from build123d import *
from build123d.topology import SkipClean

# Parameters (mm, degrees)
SKETCH1_R                 = 1.5
BOSS_EXTRUDE1_DEPTH       = 5
BOSS_EXTRUDE3_DEPTH       = 5
SKETCH4_R                 = 2.5
CUT_EXTRUDE2_DEPTH        = 5
BOSS_EXTRUDE4_DEPTH       = 5
BOSS_EXTRUDE4_2_DEPTH     = 5
BOSS_EXTRUDE5_OUTLINE_R   = 2.5
BOSS_EXTRUDE5_OUTLINE_R_2 = 1.5
BOSS_EXTRUDE5_DEPTH       = 0.01
CUT_EXTRUDE3_DEPTH        = 10
SKETCH10_R                = 1.5
CUT_EXTRUDE4_DEPTH        = 10


# Read off the part's stored shape, not the designer's step: Boss-Extrude5
with BuildPart() as part:
    # Sketch1 → Boss-Extrude1 (new body)
    with BuildSketch(Plane.XY):
        with BuildLine():
            Line((0, -4), (-70.14, -4))
            ThreePointArc((-70.14, -4), (-74.14, 0), (-70.14, 4))
            Line((-70.14, 4), (0, 4))
            ThreePointArc((0, 4), (4, 0), (0, -4))
        make_face()
        with Locations((-70.14, 0)):
            Circle(SKETCH1_R, mode=Mode.SUBTRACT)
        Circle(SKETCH1_R, mode=Mode.SUBTRACT)
    extrude(amount=BOSS_EXTRUDE1_DEPTH)

    # Sketch3 → Boss-Extrude3 (add)
    with BuildSketch(Plane.XY):
        with BuildLine():
            Line((-70.14, -4), (-77.64, -4))
            ThreePointArc((-77.64, -4), (-81.64, 0), (-77.64, 4))
            Line((-77.64, 4), (-70.14, 4))
            ThreePointArc((-70.14, 4), (-66.14, 0), (-70.14, -4))
        make_face()
    extrude(amount=BOSS_EXTRUDE3_DEPTH)

    # Sketch4 → Cut-Extrude2 (cut)
    with BuildSketch(Plane(origin=(0, 0, 0), x_dir=(-1, 0, 0), z_dir=(0, 0, -1))):
        with Locations((70.14, 0)):
            Circle(SKETCH4_R)
    extrude(amount=-CUT_EXTRUDE2_DEPTH, mode=Mode.SUBTRACT)



with BuildPart() as body_2:
    # Sketch5 → Boss-Extrude4 (new body)
    with BuildSketch(Plane.XY.offset(5)):
        with BuildLine():
            add(Edge.make_bspline(
                [(-77.64, -4), (-63.527561679, -4), (-37.041969255, -17.709059975), (-15.820527041, -4), (0, -4)],
                knots=[0, 0, 0, 0, 0.514247309, 1, 1, 1, 1], degree=3))
            Line((0, -4), (-77.64, -4))
        make_face()
    extrude(amount=-BOSS_EXTRUDE4_DEPTH)


with BuildPart() as body_3:
    # Sketch5 → Boss-Extrude4 2 (new body)
    with BuildSketch(Plane.XY.offset(5)):
        with BuildLine():
            add(Edge.make_bspline(
                [(-77.64, 4), (-63.527561679, 4), (-37.041969255, 17.709059975), (-15.820527041, 4), (0, 4)],
                knots=[0, 0, 0, 0, 0.514247309, 1, 1, 1, 1], degree=3))
            Line((0, 4), (-77.64, 4))
        make_face()
    extrude(amount=-BOSS_EXTRUDE4_2_DEPTH)


with BuildPart() as part_1:
    with SkipClean():  # the faces are left unmerged after this step: merging them gives an invalid solid
        add(part.part)

        add(body_2.part)  # Boss-Extrude5 merges body 2

        add(body_3.part)  # Boss-Extrude5 merges body 3
        # Boss-Extrude5 outline → Boss-Extrude5 (add)
        # profile 1 of 3: a face of its own
        with BuildSketch(Plane.XY.offset(5)):
            with BuildLine():
                add(Edge.make_bspline(
                    [(0, 4), (-15.820527041, 4), (-37.041969255, 17.709059975), (-63.527561679, 4), (-77.64, 4)],
                    knots=[0, 0, 0, 0, 0.485752691, 1, 1, 1, 1], degree=3))
                Line((-77.64, 4), (0, 4))
            make_face()
        # profile 2 of 3: a face of its own
        with BuildSketch(Plane.XY.offset(5)):
            with BuildLine():
                Line((0, 4), (-77.64, 4))
                ThreePointArc((-77.64, 4), (-81.64, 0), (-77.64, -4))
                Line((-77.64, -4), (0, -4))
                ThreePointArc((0, -4), (4, 0), (0, 4))
            make_face()
            with Locations((-70.14, 0)):
                Circle(BOSS_EXTRUDE5_OUTLINE_R, mode=Mode.SUBTRACT)
            Circle(BOSS_EXTRUDE5_OUTLINE_R_2, mode=Mode.SUBTRACT)
        # profile 3 of 3: a face of its own
        with BuildSketch(Plane.XY.offset(5)):
            with BuildLine():
                Line((0, -4), (-77.64, -4))
                add(Edge.make_bspline(
                    [(-77.64, -4), (-63.527561679, -4), (-37.041969255, -17.709059975), (-15.820527041, -4), (0, -4)],
                    knots=[0, 0, 0, 0, 0.514247309, 1, 1, 1, 1], degree=3))
            make_face()
        extrude(amount=BOSS_EXTRUDE5_DEPTH)
    add(part_1.part.scale(1), mode=Mode.REPLACE)  # the faces are merged on a copy

    # Sketch9 → Cut-Extrude3 (cut)
    with BuildSketch(Plane.XY.offset(5.01)):
        with BuildLine():
            add(Edge.make_bspline(
                [(-0.876672038, 4.006820197), (-16.204235996, 4.245362878), (-35.408867191, 16.400266247), (-58.905371653, 6.201116002), (-70.440504523, 4.548002129)],
                knots=[0.009030481, 0.009030481, 0.009030481, 0.009030481, 0.485752691, 0.911971345, 0.911971345, 0.911971345, 0.911971345], degree=3))
            Line((-70.440504523, 4.548002129), (-70.104638549, 4.545389211))
            Line((-70.104638549, 4.545389211), (-0.876672038, 4.006820197))
        make_face()
        with BuildLine():
            Line((0, 4), (-0.876672038, 4.006820197))
            add(Edge.make_bspline(
                [(0, 4), (-0.294114625, 4), (-0.586324171, 4.002301517), (-0.876672038, 4.006820197)],
                knots=[0, 0, 0, 0, 0.009030481, 0.009030481, 0.009030481, 0.009030481], degree=3))
        make_face()
    extrude(amount=-CUT_EXTRUDE3_DEPTH, mode=Mode.SUBTRACT)

    # Sketch10 → Cut-Extrude4 (cut)
    with BuildSketch(Plane.XY.offset(5.01)):
        with Locations((-77.14, 0)):
            Circle(SKETCH10_R)
        with Locations((-63.14, 0)):
            Circle(SKETCH10_R)
    extrude(amount=-CUT_EXTRUDE4_DEPTH, mode=Mode.SUBTRACT)


solid = part_1.part
Design review of the part built by this model. Coordinates are the model's own, in mm. Coordinates: 2 decimals unless noted, no trailing zeros. Loops run counter-clockwise (first coordinate to the right, second up) from the corner with the lowest first, then second, coordinate; pieces in that order, holes last.
Item 1: Wall thickness on L1, parallel to Y at x = -77.14, z = 2.25; L2, parallel to Y at x = -63.14, z = 3.9; L3, parallel to X at y = -0.25, z = 0.95: over which ranges is each line inside the solid? List them lowest first.
Completed:
L1: y = -4 to -1.5, 1.5 to 4
L2: y = -5.95 to -1.5, 1.5 to 4.49
L3: x = -81.63 to -78.62, -75.66 to -72.63, -67.65 to -64.62, -61.66 to -1.48, 1.48 to 3.99
Item 2: Draft analysis for pull direction Y (two halves, no side actions). For faces 1 (the cylindrical face through (4, 0, 2)), 2 (the cylindrical face through (-78.64, 0.07, 2.54)), 3 (the flat face through (-39, -1, 5.01)), state which applies: pulls with the +Y half, pulls with the -Y half, needs draft (parallel to the pull), parting line crosses it, or undercut.
Completed:
face 1: parting line crosses it
face 2: undercut
face 3: needs draft
Item 3: Clearance check with a flat-ended pin moving along its axis: pin 1 (2.5 mm diameter, centred on x = -63.14, y = 0, fed in from +Z). State where the tip first meets the part, or that it passes through.
Completed:
pin 1: passes through
Item 4: Add section A-A (y = 0). Write out the cut boundary in (x, z).
Completed:
outline: (-81.64, 0) - (-78.64, 0) - (-78.64, 5.01) - (-81.64, 5.01) - close; (-75.64, 0) - (-72.64, 0) - (-72.64, 5.01) - (-75.64, 5.01) - close; (-67.64, 0) - (-64.64, 0) - (-64.64, 5.01) - (-67.64, 5.01) - close; (-61.64, 0) - (-1.5, 0) - (-1.5, 5.01) - (-61.64, 5.01) - close; (1.5, 0) - (4, 0) - (4, 5.01) - (1.5, 5.01) - close
Item 5: Add section B-B (z = 2.8). Give the number of separate pieces and of enclosed holes in the cut face, and give its area (3 significant figures).
Completed:
separate pieces: 1
enclosed holes: 4
area: 905 mm2
